Work out the finished part from the listing and answer in its coordinate system (mm). Face numbers are marked on the shaded views. A direction names the side the tool comes from. Coordinates: 2 decimals unless noted, no trailing zeros. Order: outer loops, then holes, each group sorted by start corner. A loop starts at its lowest first (then second) coordinate and runs counter-clockwise, first axis right, second up.
1. A tool of negligible diameter and unlimited length cuts with its end or side. For the marked faces 1, 2, 3, 4 and 5, from which of +Z, -Z, +X, -X, +Y, -Y can it reach the whole face along a straight path? Write none if from no direction.
2. The part is cut by section C-C, the plane y = 11.5. Give the vertices of the cut face in (x, z).
3. Flat-ended cylindrical pins translate along their axes: pin 1 Ø3 at (x, y) = (0, 20) entering from -Z; pin 2 Ø1.5 at (x, z) = (-7, 1) entering from +Y; pin 3 Ø8 at (y, z) = (-7, 0.5) entering from +X; pin 4 Ø5 at (x, y) = (-1, -5) entering from +Z. Find the tip coordinate at first contact, or state that the pin passes through.
4. Determine the mould class of the marked faces 6, 7 and 8 for opening direction Z: +Z half, -Z half, draft (parallel to the pull), parting line (faces both ways), or undercut.
5. The part is cut by section D-D, the plane y = 22. Give the vertices of the cut face in (x, z).
6. The part is cut by section A-A, the plane x = 0. Give the vertices of the cut face in (y, z).
7. Find the intervals of material crossed by probe 1 along Y at (x, z) = (0, -8.5); probe 2 along Z at (x, y) = (0.5, 17); probe 3 along Y at (x, z) = (-4.5, 6.5), in increasing order.
8. The part is cut by section B-B, the plane z = 3.5. Give the vertices of the cut face in (x, y), then the cut area to 3 significant figures.
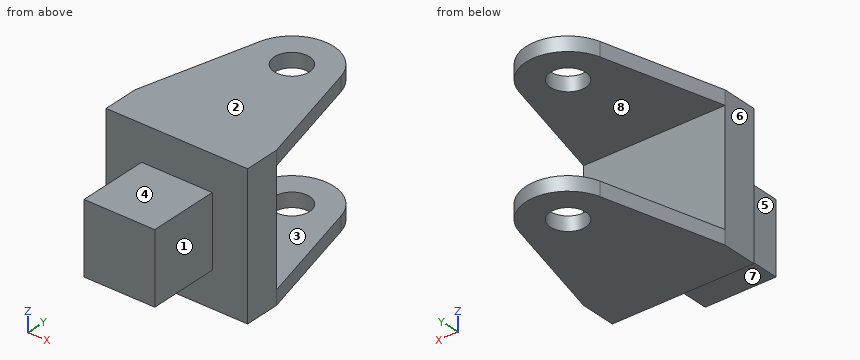
```python
from build123d import *

# Parameters (mm, degrees)
SKETCH3_W           = 20
SKETCH3_H           = 20
BOSS_EXTRUDE1_DEPTH = 30
SKETCH4_W           = 16
SKETCH4_H           = 25
CUT_EXTRUDE1_DEPTH  = 26
SKETCH7_R           = 2.5
CUT_EXTRUDE2_DEPTH  = 16.5
CUT_EXTRUDE3_DEPTH  = 33
SKETCH9_W           = 10
SKETCH9_H           = 10
BOSS_EXTRUDE2_DEPTH = 10


with BuildPart() as part:
    # Sketch3 → Boss-Extrude1 (new body)
    with BuildSketch(Plane(origin=(0, 0, 0), x_dir=(1, 0, 0), z_dir=(0, 1, 0))):
        Rectangle(SKETCH3_W, SKETCH3_H)
    extrude(amount=BOSS_EXTRUDE1_DEPTH)

    # Sketch4 → Cut-Extrude1 (cut)
    with BuildSketch(Plane.ZY.offset(10)):
        with Locations((0, 17.5)):
            Rectangle(SKETCH4_W, SKETCH4_H)
    extrude(amount=-CUT_EXTRUDE1_DEPTH, mode=Mode.SUBTRACT)

    # Sketch7 → Cut-Extrude2 (cut, symmetric)
    with BuildSketch(Plane.XY):
        with Locations((0, 20)):
            Circle(SKETCH7_R)
    extrude(amount=CUT_EXTRUDE2_DEPTH, both=True, mode=Mode.SUBTRACT)

    # Sketch8 → Cut-Extrude3 (cut)
    with BuildSketch(Plane.XY.offset(10)):
        with BuildLine():
            Line((-10, 5), (-5.739080816, 21.483527122))
            ThreePointArc((-5.739080816, 21.483527122), (0, 25.927723116), (5.739080816, 21.483527122))
            Line((5.739080816, 21.483527122), (10, 5))
            Line((10, 5), (10, 30))
            Line((10, 30), (-10, 30))
            Line((-10, 30), (-10, 5))
        make_face()
    extrude(amount=-CUT_EXTRUDE3_DEPTH, mode=Mode.SUBTRACT)

    # Sketch9 → Boss-Extrude2 (add)
    with BuildSketch(Plane.XZ):
        Rectangle(SKETCH9_W, SKETCH9_H)
    extrude(amount=BOSS_EXTRUDE2_DEPTH)


solid = part.part
```
Geometry says:
1. face 1: +Z, -Z, +X, -Y
1. face 2: +Z, +X, -X, +Y, -Y
1. face 3: +X, -X, +Y
1. face 4: +Z, +X, -X, -Y
1. face 5: +Z, -Z, -X, -Y
2. outline: (-8.32, -10) - (8.32, -10) - (8.32, -8) - (-8.32, -8) - close; (-8.32, 8) - (8.32, 8) - (8.32, 10) - (-8.32, 10) - close
3. pin 1: passes through
3. pin 2: stops at y = 5
3. pin 3: stops at x = 5
3. pin 4: stops at z = 5
4. face 6: draft
4. face 7: -Z half
4. face 8: undercut
5. outline: (-5.58, -10) - (-1.5, -10) - (-1.5, -8) - (-5.58, -8) - close; (-5.58, 8) - (-1.5, 8) - (-1.5, 10) - (-5.58, 10) - close; (1.5, -10) - (5.58, -10) - (5.58, -8) - (1.5, -8) - close; (1.5, 8) - (5.58, 8) - (5.58, 10) - (1.5, 10) - close
6. outline: (-10, -5) - (0, -5) - (0, -10) - (17.5, -10) - (17.5, -8) - (5, -8) - (5, 8) - (17.5, 8) - (17.5, 10) - (0, 10) - (0, 5) - (-10, 5) - close; (22.5, -10) - (25.93, -10) - (25.93, -8) - (22.5, -8) - close; (22.5, 8) - (25.93, 8) - (25.93, 10) - (22.5, 10) - close
7. probe 1: y = 0 to 17.5, 22.5 to 25.93
7. probe 2: z = -10 to -8, 8 to 10
7. probe 3: y = 0 to 5
8. outline: (-10, 0) - (-5, 0) - (-5, -10) - (5, -10) - (5, 0) - (10, 0) - (10, 5) - (-10, 5) - close
8. area: 200 mm2
